Work out the finished part from the listing and answer in its coordinate system (mm). A direction names the side the tool comes from. Round coordinates to 2 decimals unless told otherwise and drop trailing zeros. Write each loop counter-clockwise with the first axis right and the second up, starting at its lowest first coordinate (ties: lowest second). Pieces come first, ordered by that corner, then holes. Notation, with made-up numbers: M 4.5,59.25 L 41.5,59.25 A14 ccw 41.5,71.25 Z; hole C 86,1.25 d8. An arc over 180 degrees is marked long. One line per item, written item: value. Start each with the question number.
Q1. Consider probe 1 along X at (y, z) = (-23, -20.5); probe 2 along Z at (x, y) = (-8, 0); probe 3 along X at (y, z) = (10, -1.5). Determine where each line is inside the solid, lowest interval first.
Q2. Given pin 1 Ø2 at (y, z) = (-10, -3) entering from -X; pin 2 Ø12 at (x, y) = (9, -27.5) entering from +Z; pin 3 Ø12 at (y, z) = (2, 13.5) entering from +X; pin 4 Ø2 at (x, z) = (-31, -14) entering from +Y, each flat-ended and moving along its own axis, determine where each tip first touches the part or whether it passes through.
Q3. Find section B-B (x = -29.5). Write down the section's boundary in (y, z).
Q4. Find section C-C (z = 0). Write down the section's boundary in (x, y), and give its area (4 significant figures).
Q5. The mould has two halves that part along X. Classify faces 1 (the flat face through (1, -23.5, 0)), 2 (the cylindrical face through (52.22, -28.38, -13.62)), 3 (the flat face through (-54.5, -22, 0)): released by +X, released by -X, zero draft, split by the parting line, or undercut.
Q6. A tool of negligible diameter and unlimited length cuts with its end or side. For faces 4 (the flat face through (50, -22, -15)), 5 (the cylindrical face through (-41.06, -18.99, 0.56)), 6 (the cylindrical face through (15.8, -18.99, 0.56)), 7 (the flat face through (52.28, -28.7, 7.54)), 8 (the flat face through (-50, -22, 17)), from which of +Z, -Z, +X, -X, +Y, -Y can it reach the whole face along a straight path? Write none if from no direction.
Q7. Find section A-A (y = 0). Write down the section's boundary in (x, z), and give its area (3 significant figures).
from build123d import *

# Parameters (mm, degrees)
BOSS_EXTRUDE1_START = -24
SKETCH4_R           = 19
BOSS_EXTRUDE1_DEPTH = 4
SKETCH5_R           = 3
BOSS_EXTRUDE2_DEPTH = 54.5
CUT_EXTRUDE1_DEPTH  = 50
CHAMFER1_SIZE       = 4


with BuildPart() as part:
    # Sketch4 → Boss-Extrude1 (new body)
    with BuildSketch(Plane(origin=(0, 0, 0), x_dir=(0, 0, -1), z_dir=(1, 0, 0)).offset(BOSS_EXTRUDE1_START)):
        Circle(SKETCH4_R)
    extrude(amount=-BOSS_EXTRUDE1_DEPTH)

    # Sketch5 → Boss-Extrude2 (add, symmetric)
    with BuildSketch(Plane(origin=(0, 0, 0), x_dir=(0, 0, -1), z_dir=(1, 0, 0))):
        with BuildLine():
            Line((16.454482672, 9.5), (23.5, 9.5))
            Line((23.5, 9.5), (23.5, -34.051836095))
            Line((23.5, -34.051836095), (12.893398282, -34.051836095))
            Line((12.893398282, -34.051836095), (2.341562187, -23.5))
            Line((2.341562187, -23.5), (-2.341562187, -23.5))
            Line((-2.341562187, -23.5), (-12.893398282, -34.051836095))
            Line((-12.893398282, -34.051836095), (-23.5, -34.051836095))
            Line((-23.5, -34.051836095), (-23.5, 9.5))
            Line((-23.5, 9.5), (-16.454482672, 9.5))
            ThreePointArc((-16.454482672, 9.5), (0, -19), (16.454482672, 9.5))
        make_face()
        with Locations((16, -26.551836095)):
            Circle(SKETCH5_R, mode=Mode.SUBTRACT)
        with Locations(Location((-16, -26.551836095, 0), (0, 0, 180))):
            Circle(SKETCH5_R, mode=Mode.SUBTRACT)
    extrude(amount=BOSS_EXTRUDE2_DEPTH, both=True)

    # Sketch6 → Cut-Extrude1 (cut, symmetric)
    with BuildSketch(Plane(origin=(0, 0, 0), x_dir=(0, 0, -1), z_dir=(1, 0, 0))):
        Polygon((2.341562187, -23.5), (7.969107928, -23.5), (23.5, -10.468034191), (23.5, -34.051836095), (-23.5, -34.051836095), (-23.5, -10.468034191), (-7.969107928, -23.5), (-2.341562187, -23.5), align=None)
    extrude(amount=CUT_EXTRUDE1_DEPTH, both=True, mode=Mode.SUBTRACT)

    # Chamfer1
    chamfer1_edges = [part.edges().sort_by_distance(p)[0] for p in [
        (52.25, -34.051836095, 23.5),
        (52.25, -34.051836095, -23.5),
        (-52.25, -34.051836095, -23.5),
        (-52.25, -34.051836095, 23.5),
    ]]
    chamfer(chamfer1_edges, length=CHAMFER1_SIZE)


solid = part.part
The answers:
1. probe 1: -54.5 to -50, 50 to 54.5
1. probe 2: -23.5 to -19, 19 to 23.5
1. probe 3: -28 to -24
2. pin 1: x = -28
2. pin 2: z = 10.35
2. pin 3: x = 54.5
2. pin 4: y = -11.66
3. outline: M -23.5,-7.97 L -10.47,-23.5 L 9.5,-23.5 L 9.5,-16.45 A19 cw long 9.5,16.45 L 9.5,23.5 L -10.47,23.5 L -23.5,7.97 Z
4. outline: M -54.5,-23.5 L 54.5,-23.5 L 54.5,-19 L -24,-19 L -24,19 L -28,19 L -28,-19 L -54.5,-19 Z
4. area: 642.5 mm2
5. face 1: undercut
5. face 2: zero draft
5. face 3: released by -X
6. face 4: -Z, -Y
6. face 5: -X
6. face 6: +X
6. face 7: +X, -X, -Y
6. face 8: +Z, -Y
7. outline: M -54.5,-23.5 L 54.5,-23.5 L 54.5,-19 L -24,-19 L -24,19 L 54.5,19 L 54.5,23.5 L -54.5,23.5 L -54.5,19 L -28,19 L -28,-19 L -54.5,-19 Z
7. area: 1,130 mm2
